The drawing under review shows one solid part. Ordinate dimensions are in mm from its lowest x, y, z. Coordinates: 2 decimals unless noted, no trailing zeros. Loops run counter-clockwise (first coordinate to the right, second up) from the corner with the lowest first, then second, coordinate; pieces in that order, holes last. Notation, with made-up numbers: M 57,-6.5 L 115,-6.5 A14 cw 115,12.5 Z; hole C 32.25,30 d8. An arc over 180 degrees is marked long. Put each result on its own line as item: value.
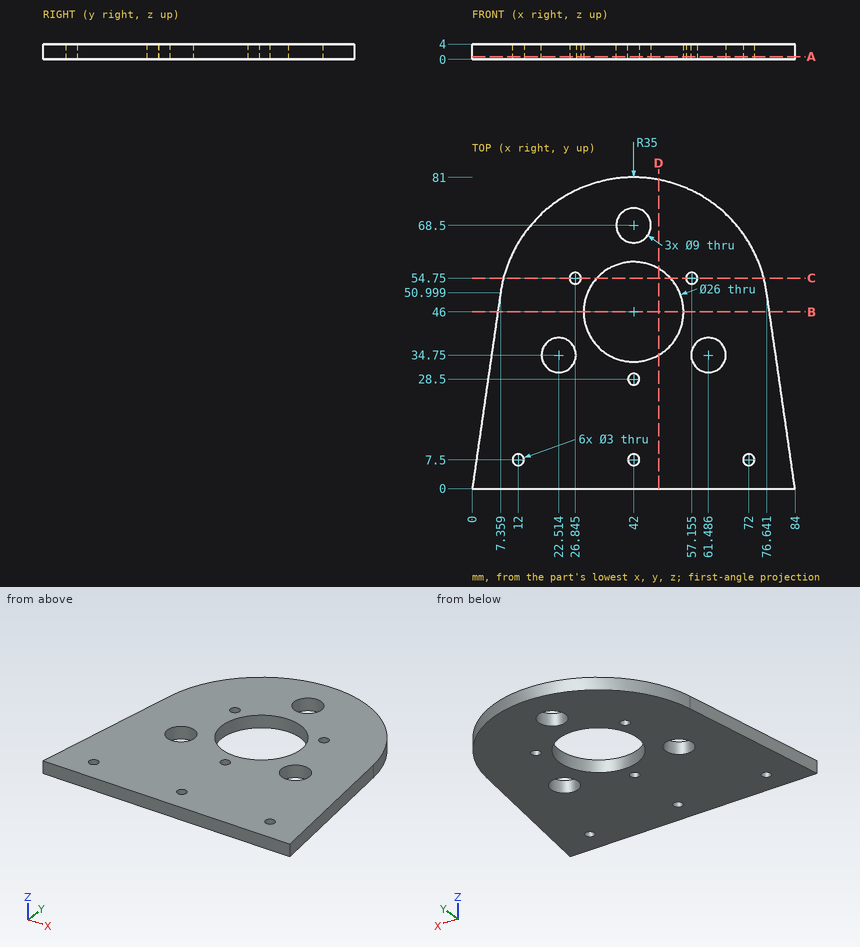
(1) Add section C-C (y = 54.75). Write out the cut boundary in (x, z) (1 decimal), plus the area to 3 significant figures.
Determined:
outline: M 8.1,0 L 25.3,0 L 25.3,4 L 8.1,4 Z; M 28.3,0 L 32.4,0 L 32.4,4 L 28.3,4 Z; M 51.6,0 L 55.7,0 L 55.7,4 L 51.6,4 Z; M 58.7,0 L 75.9,0 L 75.9,4 L 58.7,4 Z
area: 170 mm^2
(2) Wall thickness on line 1 along Y through (x, z) = (42.5, 0.55) (1 decimal); line 2 along X through (y, z) = (70, 0.4) (1 decimal); line 3 along X through (y, z) = (52.5, 3.65): over which ranges is each line inside the solid? List them lowest first. Write a range as [from, to].
Determined:
line 1: y = [0, 6.1], [8.9, 27.1], [29.9, 33], [59, 64], [73, 81]
line 2: x = [16.5, 37.8], [46.2, 67.5]
line 3: x = [7.61, 30.74], [53.26, 76.39]
(3) Add section B-B (y = 46). Write out the cut boundary in (x, z).
Determined:
outline: M 6.64,0 L 29,0 L 29,4 L 6.64,4 Z; M 55,0 L 77.36,0 L 77.36,4 L 55,4 Z
(4) For pin 1 (2 mm diameter, centred on x = 31.5, z = 0.5, fed in from +Y), flat-tipped, find the tip position at first contact; note if it passes through.
Determined:
pin 1: stops at y = 79.69
(5) Add section D-D (x = 48.5). Write out the cut boundary in (y, z).
Determined:
outline: M 0,0 L 34.74,0 L 34.74,4 L 0,4 Z; M 57.26,0 L 80.39,0 L 80.39,4 L 57.26,4 Z
(6) Add section A-A (z = 0.7). State how many separate pieces and enclosed holes the cut face has, plus the area to 3 significant figures.
Determined:
separate pieces: 1
enclosed holes: 10
area: 4,720 mm^2
